Part model, mm, in its own coordinate system. Round coordinates to 2 decimals unless told otherwise and drop trailing zeros. Loops run counter-clockwise (first coordinate to the right, second up) from the corner with the lowest first, then second, coordinate; pieces in that order, holes last.
1) Band-saw the part on B-B, the plane x = 59. Write the cut outline in (y, z), then the cut area to 3 significant figures.
2) Probe line 1 (Z direction, x = -3, y = 0.5); line 2 (X direction, y = 1.6, z = -7). List the from-to ranges inside material, lowest first.
3) Drop flat-ended pins along their axis: P1, Ø1.3, axis at x = -31.5, y = 1.5, coming from the -Z side; P2, Ø0.8, axis at y = 1.5, z = -11.5, coming from the +X side; P3, Ø1.3, axis at x = -32.5, y = 1.5, coming from the +Z side; P4, Ø2, axis at x = 59.5, z = -11, coming from the -Y side. Give the stop position or say it passes through.
4) Band-saw the part on A-A, the plane z = 6.5. Write the cut outline in (x, y), then the cut area to 3 significant figures.
from build123d import *

# Parameters (mm, degrees)
SKETCH1_W           = 144.78
SKETCH1_H           = 48.006
BOSS_EXTRUDE1_DEPTH = 2.54
SKETCH2_OUTSIDE_W   = 177.29
SKETCH2_OUTSIDE_H   = 80.516
CUT_EXTRUDE1_DEPTH  = 2.54


with BuildPart() as part:
    # Sketch1 → Boss-Extrude1 (new body)
    with BuildSketch(Plane(origin=(0, 0, 0), x_dir=(1, 0, 0), z_dir=(0, 1, 0))):
        with Locations((2.921, 0)):
            Rectangle(SKETCH1_W, SKETCH1_H)
    extrude(amount=BOSS_EXTRUDE1_DEPTH)

    # Sketch2 outside → Cut-Extrude1 (cut)
    with BuildSketch(Plane(origin=(0, 2.54, 0), x_dir=(1, 0, 0), z_dir=(0, 1, 0))):
        with Locations((2.921, 0)):
            Rectangle(SKETCH2_OUTSIDE_W, SKETCH2_OUTSIDE_H)
        Polygon((-69.469, 24.003), (-69.469, 14.4018), (-66.929, 14.4018), (-66.929, 4.8006), (-69.469, 4.8006), (-69.469, -4.8006), (-66.929, -4.8006), (-66.929, -14.4018), (-69.469, -14.4018), (-69.469, -24.003), (-58.332076923, -24.003), (-58.332076923, -21.463), (-47.195153846, -21.463), (-47.195153846, -24.003), (-36.058230769, -24.003), (-36.058230769, -21.463), (-24.921307692, -21.463), (-24.921307692, -24.003), (-13.784384615, -24.003), (-13.784384615, -21.463), (-2.647461538, -21.463), (-2.647461538, -24.003), (8.489461538, -24.003), (8.489461538, -21.463), (19.626384615, -21.463), (19.626384615, -24.003), (30.763307692, -24.003), (30.763307692, -21.463), (41.900230769, -21.463), (41.900230769, -24.003), (53.037153846, -24.003), (53.037153846, -21.463), (64.174076923, -21.463), (64.174076923, -24.003), (75.311, -24.003), (75.311, -14.4018), (72.771, -14.4018), (72.771, -4.8006), (75.311, -4.8006), (75.311, 4.8006), (72.771, 4.8006), (72.771, 14.4018), (75.311, 14.4018), (75.311, 24.003), (64.174076923, 24.003), (64.174076923, 21.463), (53.037153846, 21.463), (53.037153846, 24.003), (41.900230769, 24.003), (41.900230769, 21.463), (30.763307692, 21.463), (30.763307692, 24.003), (19.626384615, 24.003), (19.626384615, 21.463), (8.489461538, 21.463), (8.489461538, 24.003), (-2.647461538, 24.003), (-2.647461538, 21.463), (-13.784384615, 21.463), (-13.784384615, 24.003), (-24.921307692, 24.003), (-24.921307692, 21.463), (-36.058230769, 21.463), (-36.058230769, 24.003), (-47.195153846, 24.003), (-47.195153846, 21.463), (-58.332076923, 21.463), (-58.332076923, 24.003), align=None, mode=Mode.SUBTRACT)
    extrude(amount=-CUT_EXTRUDE1_DEPTH, mode=Mode.SUBTRACT)


solid = part.part
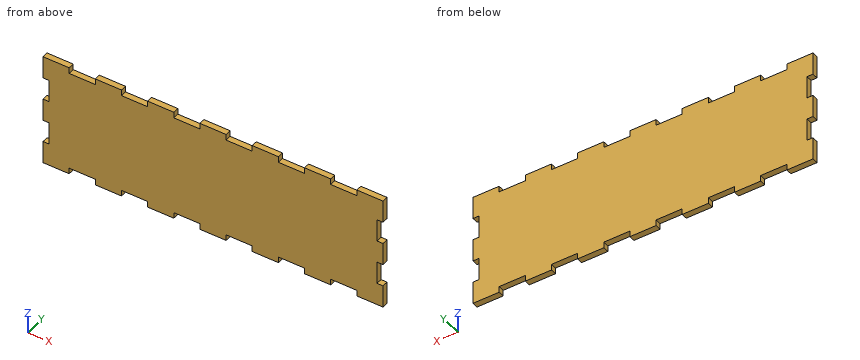
Reported:
1. outline: (0, -21.46) - (2.54, -21.46) - (2.54, 21.46) - (0, 21.46) - close
1. area: 109 mm2
2. line 1: z = -21.46 to 21.46
2. line 2: x = -66.93 to 72.77
3. P1: stops at z = -21.46
3. P2: stops at x = 72.77
3. P3: stops at z = 21.46
3. P4: stops at y = 0
4. outline: (-66.93, 0) - (72.77, 0) - (72.77, 2.54) - (-66.93, 2.54) - close
4. area: 355 mm2
